For this review, use the dimensioned drawing (mm, ordinates from the lowest corner) and the shaded views. Coordinates: 2 decimals unless noted, no trailing zeros. Write each loop counter-clockwise with the first axis right and the second up, starting at its lowest first coordinate (ties: lowest second). Pieces come first, ordered by that corner, then holes. Notation, with made-up numbers: (56.25, 83.5) - (99.25, 83.5) arc R15 ccw to (99.25, 89.5) - close; hole circle Ø10 at (8, -35.5). An arc over 180 degrees is marked (long way). One line per item, written item: value.
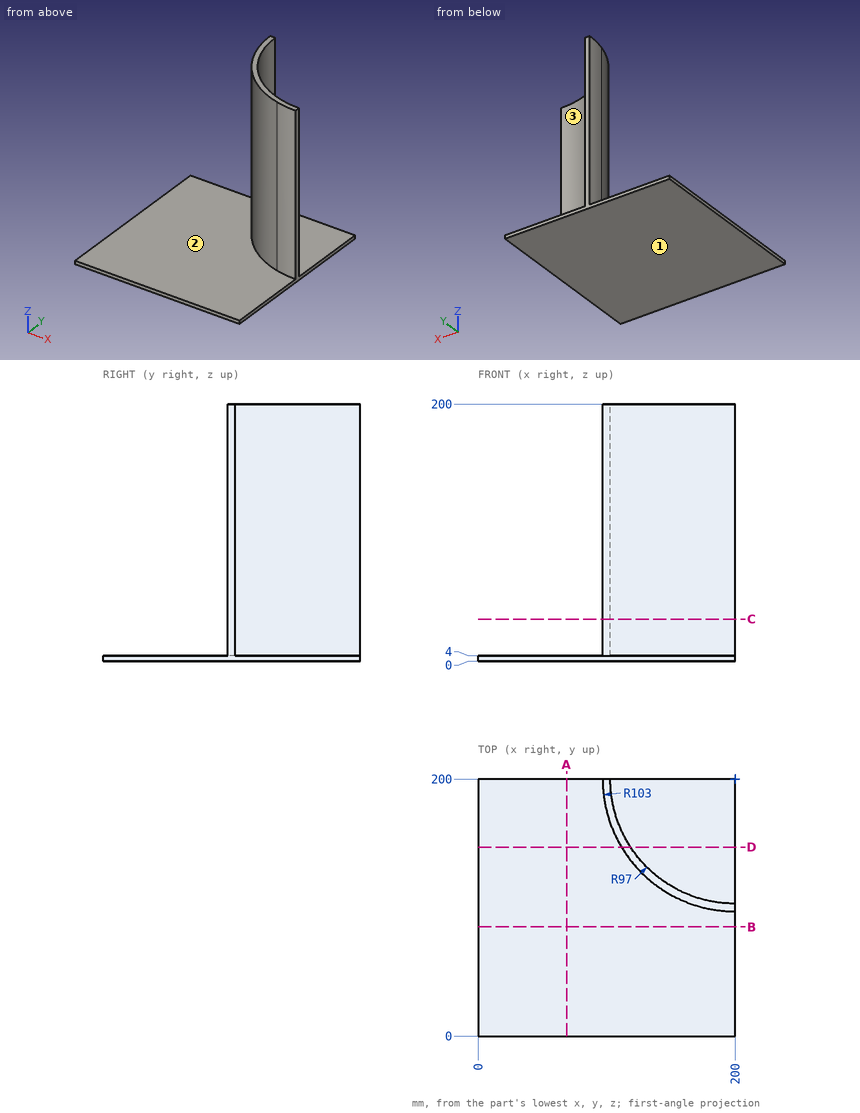
1. Wall thickness on line 1 along Z through (x, y) = (140, 88.5); line 2 along X through (y, z) = (173, 172); line 3 along Y through (x, z) = (120, 95): over which ranges is each line inside the solid? List them lowest first.
Answer block:
line 1: z = 0 to 4
line 2: x = 100.6 to 106.83
line 3: y = 135.12 to 145.15
2. Mouldability with a two-part tool opening along Z and no side actions: class the marked faces 1, 2 and 3 as released by +Z, released by -Z, zero draft, split by the parting line, or undercut.
Answer block:
face 1: released by -Z
face 2: released by +Z
face 3: zero draft
3. Insertion check: pin 1 Ø12 at (y, z) = (132, 120.5) entering from +X; pin 2 Ø2 at (y, z) = (164, 61) entering from +X; pin 3 Ø1 at (x, y) = (113.5, 58) entering from +Z. Each pin has a flat end and moves straight along its axis. Give the tip position at first contact, or say it passes through.
Answer block:
pin 1: stops at x = 137.29
pin 2: stops at x = 110.33
pin 3: stops at z = 4
4. Consider section C-C, the plane z = 32.5. Write out the cut boundary in (x, y), then the cut area to 3 significant figures.
Answer block:
outline: (97, 200) arc R103 ccw to (200, 97) - (200, 103) arc R97 cw to (103, 200) - close
area: 942 mm^2
5. Consider section D-D, the plane y = 147. Write out the cut boundary in (x, z).
Answer block:
outline: (0, 0) - (200, 0) - (200, 4) - (118.76, 4) - (118.76, 200) - (111.68, 200) - (111.68, 4) - (0, 4) - close
6. Consider section A-A, the plane x = 69. Write out the cut boundary in (y, z), then the cut area to 3 significant figures.
Answer block:
outline: (0, 0) - (200, 0) - (200, 4) - (0, 4) - close
area: 800 mm^2
